from build123d import *

# Parameters (mm, degrees)
CROQUIS1_W                 = 72.3
CROQUIS1_H                 = 65.58
SALIENTE_EXTRUIR1_DEPTH    = 35.75
CROQUIS2_R                 = 12
CORTAR_EXTRUIR1_DEPTH      = 2
CROQUIS3_R                 = 17.5
CROQUIS3_R_2               = 3
CORTAR_EXTRUIR2_DEPTH      = 10
CORTAR_EXTRUIR3_DEPTH      = 61.49850494
CORTAR_EXTRUIR3_DEPTH_BACK = 61.49850494
CORTAR_EXTRUIR4_DEPTH      = 31
CROQUIS3_3_R               = 3.175
CORTAR_EXTRUIR5_DEPTH      = 83.979644492
CORTAR_EXTRUIR6_DEPTH      = 83.979644492


with BuildPart() as part:
    # Croquis1 → Saliente-Extruir1 (new, symmetric)
    with BuildSketch(Plane(origin=(0, 0, 0), x_dir=(1, 0, 0), z_dir=(0, 1, 0))):
        Rectangle(CROQUIS1_W, CROQUIS1_H)
    extrude(amount=SALIENTE_EXTRUIR1_DEPTH, both=True)

    # Croquis2 → Cortar-Extruir1 (cut)
    # profile 1 of 3: a face of its own
    with BuildSketch(Plane(origin=(36.15, 0, 0), x_dir=(0, 0, -1), z_dir=(1, 0, 0))):
        Polygon((-20.6, 20.466990028), (-20.6, 35.75), (-32.79, 35.75), (-32.79, -35.75), (-20.6, -35.75), (-20.6, -24.184428132), (-20.6, -12.075571868), (-20.6, -0.51), (-20.6, 0.27), (-20.6, 15.553009972), align=None)
    # profile 2 of 3: a face of its own
    with BuildSketch(Plane(origin=(36.15, 0, 0), x_dir=(0, 0, -1), z_dir=(1, 0, 0))):
        with BuildLine():
            Line((22.77, 35.75), (-20.6, 35.75))
            Line((-20.6, 35.75), (-20.6, 20.466990028))
            ThreePointArc((-20.6, 20.466990028), (-9.82, 18.01), (-20.6, 15.553009972))
            Line((-20.6, 15.553009972), (-20.6, 0.27))
            Line((-20.6, 0.27), (22.77, 0.27))
            Line((22.77, 0.27), (28.535, 6.035))
            Line((28.535, 6.035), (28.535, 29.985))
            Line((28.535, 29.985), (22.77, 35.75))
        make_face()
        with Locations((8.87, 18.01)):
            Circle(CROQUIS2_R, mode=Mode.SUBTRACT)
    # profile 3 of 3: a face of its own
    with BuildSketch(Plane(origin=(36.15, 0, 0), x_dir=(0, 0, -1), z_dir=(1, 0, 0))):
        with BuildLine():
            Line((-20.6, -24.184428132), (-20.6, -35.75))
            Line((-20.6, -35.75), (2.65, -35.75))
            Line((2.65, -35.75), (7.66, -30.08))
            Line((7.66, -30.08), (7.66, -6.18))
            Line((7.66, -6.18), (2.65, -0.51))
            Line((2.65, -0.51), (-20.6, -0.51))
            Line((-20.6, -0.51), (-20.6, -12.075571868))
            ThreePointArc((-20.6, -12.075571868), (1.09, -18.13), (-20.6, -24.184428132))
        make_face()
    extrude(amount=-CORTAR_EXTRUIR1_DEPTH, mode=Mode.SUBTRACT)

    # Croquis3 → Cortar-Extruir2 (cut)
    # profile 1 of 2: a face of its own
    with BuildSketch(Plane.XY.offset(32.79)):
        with BuildLine():
            Line((34.15, -25.16), (34.15, 18.25))
            Line((34.15, 18.25), (29.164563997, 18.25))
            ThreePointArc((29.164563997, 18.25), (-21.846955575, -2.732617016), (28.546078054, -25.16))
            Line((28.546078054, -25.16), (34.15, -25.16))
        make_face()
        with Locations((8.15, -3.16)):
            Circle(CROQUIS3_R, mode=Mode.SUBTRACT)
    # profile 2 of 2: a face of its own
    with BuildSketch(Plane.XY.offset(32.79)):
        with Locations((8.15, -3.16)):
            Circle(CROQUIS3_R_2)
    extrude(amount=-CORTAR_EXTRUIR2_DEPTH, mode=Mode.SUBTRACT)

    # Croquis4 → Cortar-Extruir3 (cut, two sides: drawn at the far end of the back side and taken through both)
    with BuildSketch(Plane(origin=(0, 0, 0), x_dir=(1, 0, 0), z_dir=(0, 1, 0)).offset(-CORTAR_EXTRUIR3_DEPTH_BACK)):
        Polygon((-36.15, 32.79), (23.958, 32.79), (-36.15, -20.6), align=None)
    extrude(amount=CORTAR_EXTRUIR3_DEPTH + CORTAR_EXTRUIR3_DEPTH_BACK, mode=Mode.SUBTRACT)

    # Croquis5 → Cortar-Extruir4 (cut, symmetric)
    with BuildSketch(Plane(origin=(0, 0, 0), x_dir=(1, 0, 0), z_dir=(0, 1, 0))):
        Polygon((23.958, 32.79), (23.958, -20.6), (-36.15, -20.6), align=None)
    extrude(amount=CORTAR_EXTRUIR4_DEPTH, both=True, mode=Mode.SUBTRACT)

    # Croquis3_3 → Cortar-Extruir5 (cut, through all)
    with BuildSketch(Plane.XY.offset(32.79)):
        with Locations((-24.852904541, 27.365641017)):
            Circle(CROQUIS3_3_R)
    extrude(amount=-CORTAR_EXTRUIR5_DEPTH, mode=Mode.SUBTRACT)

    # Croquis6 → Cortar-Extruir6 (cut, through all)
    with BuildSketch(Plane.XY.offset(32.79)):
        Polygon((-36.15, 32.75), (-36.15, 35.75), (34.15, 35.75), align=None)
        Polygon((-36.15, -32.75), (-36.15, -35.75), (34.15, -35.75), align=None)
    extrude(amount=-CORTAR_EXTRUIR6_DEPTH, mode=Mode.SUBTRACT)


solid = part.part
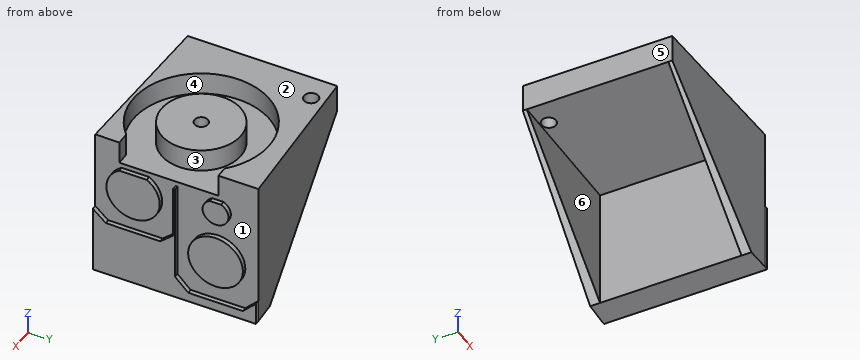
Could you check a few things on this model? Use its own coordinates, in mm. Face numbers are marked on the shaded views. A direction names the side the tool comes from. Give positions to 0.01 mm unless a question says otherwise; leave off trailing zeros. Write each loop counter-clockwise with the first axis right and the second up, starting at its lowest first coordinate (ties: lowest second). Pieces come first, ordered by that corner, then holes. Notation, with made-up numbers: (-9, -9) -> (26, -9) arc R23 cw to (26, 18) -> close; hole circle Ø5 at (36.25, 74.5). An arc over 180 degrees is marked (long way). Answer as a JSON object with one key per item and string values.
Q1. Suppose I cut it at B-B on x = -3.5. Write out the boundary of the cut face in (y, z), then the cut area to 3 significant figures.
Taken from the geometry:
{"outline": "(-34.14, -8.4) -> (-31, -8.4) -> (-31, 20.6) -> (31, 20.6) -> (31, -8.4) -> (34.14, -8.4) -> (34.14, 32.79) -> (24.49, 32.79) -> (24.49, 22.79) -> (9.9, 22.79) -> (9.9, 32.79) -> (-16.22, 32.79) -> (-16.22, 22.79) -> (-30.81, 22.79) -> (-30.81, 32.79) -> (-34.14, 32.79) -> close", "area": "723 mm²"}
Q2. Suppose I cut it at C-C on y = -17.5. Write out the boundary of the cut face in (x, z), then the cut area to 3 significant figures.
Taken from the geometry:
{"outline": "(-36.15, 20.6) -> (23.96, 20.6) -> (23.96, -32.79) -> (36.15, -32.79) -> (36.15, -7.66) -> (34.15, -7.66) -> (34.15, -1.07) -> (36.15, -1.07) -> (36.15, 20.6) -> (34.15, 20.6) -> (34.15, 22.79) -> (18.18, 22.79) -> (18.18, 32.79) -> (-1.88, 32.79) -> (-1.88, 22.79) -> (-18.2, 22.79) -> (-18.2, 32.79) -> (-36.15, 32.79) -> close", "area": "1,170 mm²"}
Q3. Suppose I cut it at A-A on z = 28. Write out the boundary of the cut face in (x, y) (3 decimals), then the cut area to 3 significant figures.
Taken from the geometry:
{"outline": "(-36.15, -32.75) -> (34.15, -35.75) -> (34.15, -25.16) -> (28.546, -25.16) arc R30 cw (long way) to (29.165, 18.25) -> (34.15, 18.25) -> (34.15, 35.75) -> (-36.15, 32.75) -> close; circle Ø35 at (8.15, -3.16); hole circle Ø6.35 at (-24.853, 27.366); hole circle Ø6 at (8.15, -3.16)", "area": "2,940 mm²"}
Q4. Will these pins go through, and if not, where does the flat tip stop? pin 1 Ø5.5 at (x, y) = (8.15, -3.16) entering from +Z; pin 2 Ø4.5 at (x, z) = (30, 28.5) entering from +Y; pin 3 Ø1.6 at (x, z) = (35, 5) entering from +Y.
Taken from the geometry:
{"pin 1": "stops at z = 22.79", "pin 2": "stops at y = 35.67", "pin 3": "stops at y = 0.27"}
Q5. We'd pull the mould along Z, two halves only. Please class the marked faces 1, 2 and 3: released by +Z, released by -Z, zero draft, split by the parting line, or undercut.
Taken from the geometry:
{"face 1": "undercut", "face 2": "released by +Z", "face 3": "zero draft"}
Q6. Please list where these lines run through material, in increasing order: L1, parallel to X at y = -3, z = 27; L2, parallel to Y at x = 8.15, z = 25.75; L3, parallel to Y at x = 22.5, z = 23.5.
Taken from the geometry:
{"L1": "x = -36.15 to -21.85, -9.35 to 5.15, 11.15 to 25.65", "L2": "y = -34.64 to -33.16, -20.66 to -6.16, -0.16 to 14.34, 26.84 to 34.64", "L3": "y = -35.25 to -29.51, -13.18 to 6.86, 23.19 to 35.25"}
Q7. Which directions (+Z, -Z, +X, -X, +Y, -Y) give clear straight access to the entire face, cutting with the end or side of a thin tool? Please do the marked faces 4, 5 and 6.
Taken from the geometry:
{"face 4": "+Z", "face 5": "+Z, -Z, -X, +Y, -Y", "face 6": "-Z, -X"}
Q8. Suppose I cut it at D-D on z = -4. Write out the boundary of the cut face in (x, y).
Taken from the geometry:
{"outline": "(-8.45, -33.93) -> (34.15, -35.75) -> (36.15, -35.75) -> (36.15, -34.22) -> (34.15, -34.22) -> (34.15, -2.04) -> (36.15, -2.04) -> (36.15, 0.27) -> (34.15, 0.27) -> (34.15, 7.04) -> (36.15, 7.04) -> (36.15, 28.98) -> (34.15, 28.98) -> (34.15, 35.75) -> (-8.45, 33.93) -> (-8.45, 31) -> (23.96, 31) -> (23.96, -31) -> (-8.45, -31) -> close"}
